Here's how the part is built. I have some questions about the finished solid (model axes, mm). A direction names the side the tool comes from. Round coordinates to 2 decimals unless told otherwise and drop trailing zeros. Write each loop counter-clockwise with the first axis right and the second up, starting at its lowest first coordinate (ties: lowest second). Pieces come first, ordered by that corner, then holes. Notation, with made-up numbers: (81.5, 24) -> (124.5, 24) arc R28 cw to (124.5, 53) -> close; hole circle Ø4 at (8, 61.5). An arc over 180 degrees is marked (long way). Put each result on its own line as item: value. Start each with the question number.
1) I want a section at A-A, the plane z = 7. List the corners of the cut face in (x, y) for me.
2) I want a section at B-B, the plane y = 0. List the corners of the cut face in (x, z) for me (3 decimals).
3) I want a section at C-C, the plane x = -3.5. List the corners of the cut face in (y, z) for me.
4) Which directions (+Z, -Z, +X, -X, +Y, -Y) give clear straight access to the entire face, cutting with the end or side of a thin tool? Please do faces 4 (the flat face through (6, -3.417, 10)), 5 (the flat face through (21.209, -7, 11)), 6 (the flat face through (14, 6.743, 3)), 7 (the flat face through (4.191, -7, 11)).
5) Will these pins go through, and if not, where does the flat tip stop? P1, Ø5, axis at x = 6, y = 1, coming from the -Z side; P2, Ø5.5, axis at y = -7.23, z = 15.24, coming from the +X side; P3, Ø7.5, axis at x = 32.39, y = -2.15, coming from the +Z side; P4, Ø4, axis at y = -5.5, z = 10, coming from the -X side.
6) If I drill on line 1 along X through (y, z) = (-7.75, 8); line 2 along Z through (x, y) = (-7.5, -6.5); line 3 along X through (y, z) = (-4, 4) (3 decimals), over which ranges is the centre line in solid material (lowest first)? Write a range as [from, to].
7) We'd pull the mould along X, two halves only. Please class faces 1 (the flat face through (8.001, -7, 11)), 2 (the cylindrical face through (-9.346, 5.215, 3.219)), 3 (the cylindrical face through (38, -10, 3)): released by +X, released by -X, zero draft, split by the parting line, or undercut.
8) I want a section at D-D, the plane z = 15.24. Give the number of separate pieces and of enclosed holes in the cut face, then the cut area to 3 significant figures.
from build123d import *

# Parameters (mm, degrees)
F0_W        = 50.8
F0_H        = 17.78
F0_R        = 3.3655
F1_DEPTH    = 6.35
F2_R        = 5.08
F3_W        = 3.81
F3_H        = 7.62
F4_DEPTH    = 12.7
F5_R        = 2.3495
F6_DEPTH    = 25.4
F7_T1_DEPTH = 26.67
F7_T3_DEPTH = 26.67


# Not quite as in the source:
# - a fillet or chamfer that OpenCascade refuses, or shapes differently, is made with other operations: its cross-section is extruded or revolved along the edge and cut away or added


with BuildPart() as f1:
    # F0 (on Top) → F1 (new body)
    with BuildSketch(Plane.XY):
        with Locations((14.6050021708, -2.1469597467)):
            Rectangle(F0_W, F0_H)
        with Locations((-3.1749978292, -2.1469597467)):
            Circle(F0_R, mode=Mode.SUBTRACT)
        with Locations((32.3850021708, -2.1469597467)):
            Circle(F0_R, mode=Mode.SUBTRACT)
    extrude(amount=F1_DEPTH)

    # F2
    f2_edges = [f1.edges().sort_by_distance(p)[0] for p in [
        (40.005002, -11.03696, 3.175),
        (40.005002, 6.74304, 3.175),
        (-10.794998, -11.03696, 3.175),
        (-10.794998, 6.74304, 3.175),
    ]]
    fillet(f2_edges, radius=F2_R)

    # F3 (on face) → F4 (join)
    with BuildSketch(Plane.XY.offset(6.35)):
        with Locations((6.0960021708, -7.2269597467)):
            Rectangle(F3_W, F3_H)
        with Locations((23.1140021708, -7.2269597467)):
            Rectangle(F3_W, F3_H)
    extrude(amount=F4_DEPTH)

    # F5 (on face) → F6 (cut)
    with BuildSketch(Plane.YZ.offset(25.0190021708)):
        with Locations((-7.2269597467, 15.24)):
            Circle(F5_R)
    extrude(amount=-F6_DEPTH, mode=Mode.SUBTRACT)

    # F7: fillet of radius 4.572 on 4 edges, made by hand

    # F7_s2 → F7_t1 (cut)
    with BuildSketch(Plane.YZ.offset(-7.2389978292)):
        with BuildLine():
            add(Edge.make_bspline(
                [(-11.0369597467, 14.478), (-11.0369597467, 19.05), (-6.4649597467, 19.05)],
                knots=[0, 0, 0, 1, 1, 1], degree=2, weights=[1, 1, 1]))
            Line((-6.4649597467, 19.05), (-11.0369597467, 19.05))
            Line((-11.0369597467, 19.05), (-11.0369597467, 14.478))
        make_face()
        with BuildLine():
            add(Edge.make_bspline(
                [(-3.4169597467, 14.478), (-3.4169597467, 19.05), (-7.9889597467, 19.05)],
                knots=[0, 0, 0, 1, 1, 1], degree=2, weights=[1, 1, 1]))
            Line((-7.9889597467, 19.05), (-3.4169597467, 19.05))
            Line((-3.4169597467, 19.05), (-3.4169597467, 14.478))
        make_face()
    extrude(amount=F7_T1_DEPTH, mode=Mode.SUBTRACT)

    # F7_s4 → F7_t3 (cut)
    with BuildSketch(Plane.YZ.offset(9.7790021708)):
        with BuildLine():
            add(Edge.make_bspline(
                [(-11.0369597467, 14.478), (-11.0369597467, 19.05), (-6.4649597467, 19.05)],
                knots=[0, 0, 0, 1, 1, 1], degree=2, weights=[1, 1, 1]))
            Line((-6.4649597467, 19.05), (-11.0369597467, 19.05))
            Line((-11.0369597467, 19.05), (-11.0369597467, 14.478))
        make_face()
        with BuildLine():
            add(Edge.make_bspline(
                [(-3.4169597467, 14.478), (-3.4169597467, 19.05), (-7.9889597467, 19.05)],
                knots=[0, 0, 0, 1, 1, 1], degree=2, weights=[1, 1, 1]))
            Line((-7.9889597467, 19.05), (-3.4169597467, 19.05))
            Line((-3.4169597467, 19.05), (-3.4169597467, 14.478))
        make_face()
    extrude(amount=F7_T3_DEPTH, mode=Mode.SUBTRACT)


solid = f1.part
Findings:
1. outline: (4.19, -11.04) -> (8, -11.04) -> (8, -3.42) -> (4.19, -3.42) -> close; (21.21, -11.04) -> (25.02, -11.04) -> (25.02, -3.42) -> (21.21, -3.42) -> close
2. outline: (-10.795, 0) -> (-5.767, 0) -> (-5.767, 6.35) -> (-10.795, 6.35) -> close; (-0.583, 0) -> (29.793, 0) -> (29.793, 6.35) -> (-0.583, 6.35) -> close; (34.977, 0) -> (40.005, 0) -> (40.005, 6.35) -> (34.977, 6.35) -> close
3. outline: (-11.04, 0) -> (-5.5, 0) -> (-5.5, 6.35) -> (-11.04, 6.35) -> close; (1.2, 0) -> (6.74, 0) -> (6.74, 6.35) -> (1.2, 6.35) -> close
4. face 4: +Z, +X, -X, +Y
4. face 5: +Z, +Y, -Y
4. face 6: +Z, -Z, +X, -X, +Y
4. face 7: +Z, -X, +Y, -Y
5. P1: stops at z = 0
5. P2: stops at x = 25.02
5. P3: stops at z = 6.35
5. P4: stops at x = 4.19
6. line 1: x = [4.19, 8], [21.21, 25.02]
6. line 2: z = [0, 6.35]
6. line 3: x = [-10.795, -5.984], [-0.366, 29.576], [35.194, 40.005]
7. face 1: undercut
7. face 2: released by -X
7. face 3: released by +X
8. separate pieces: 4
8. enclosed holes: 0
8. area: 21.7 mm2
